```python
from build123d import *

# Parameters (mm, degrees)
SKETCH1_R           = 75
BOSS_EXTRUDE1_DEPTH = 102
SKETCH3_R           = 51
BOSS_EXTRUDE2_DEPTH = 102
SKETCH4_R           = 38
BOSS_EXTRUDE3_DEPTH = 75


with BuildPart() as part:
    # Sketch1 → Boss-Extrude1 (new body)
    with BuildSketch(Plane(origin=(0, 0, 0), x_dir=(1, 0, 0), z_dir=(0, 1, 0))):
        with BuildLine():
            Line((-179.614887026, -98.810385884), (-355, 220))
            Line((-355, 220), (-355, 495))
            Line((-355, 495), (355, 495))
            Line((355, 495), (355, 220))
            Line((355, 220), (179.614887026, -98.810385884))
            ThreePointArc((179.614887026, -98.810385884), (0, -205), (-179.614887026, -98.810385884))
        make_face()
        with Locations(Location((0, 0, 0), (0, 0, 270))):
            Circle(SKETCH1_R, mode=Mode.SUBTRACT)
    boss_extrude1 = extrude(amount=BOSS_EXTRUDE1_DEPTH)

    # Sketch3 → Boss-Extrude2 (add)
    with BuildSketch(Plane(origin=(355, 0, 0), x_dir=(0, 0, -1), z_dir=(1, 0, 0))):
        with BuildLine():
            Line((220, 0), (220, 745))
            Line((220, 745), (495, 745))
            Line((495, 745), (901.007583532, 165.230354266))
            ThreePointArc((901.007583532, 165.230354266), (908.13749835, 56.5190099), (815, 0))
            Line((815, 0), (220, 0))
        make_face()
        with Locations((815, 105)):
            Circle(SKETCH3_R, mode=Mode.SUBTRACT)
    boss_extrude2 = extrude(amount=-BOSS_EXTRUDE2_DEPTH)

    # Mirror1: Boss-Extrude2 across plane
    add(boss_extrude2.mirror(Plane(origin=(0, 0, 0), x_dir=(0, 0, 1), z_dir=(1, 0, 0))))

    # Mirror2: Boss-Extrude1 across plane
    add(boss_extrude1.mirror(Plane(origin=(0, 372.5, 0), x_dir=(0, 0, 1), z_dir=(0, -1, 0))))

    # Sketch4 → Boss-Extrude3 (add)
    with BuildSketch(Plane(origin=(100, 0, 0), x_dir=(0, 0, -1), z_dir=(1, 0, 0))):
        with BuildLine():
            Line((440.558080551, 1007.850884872), (220, 745))
            Line((220, 745), (454.97331208, 745))
            Line((454.97331208, 745), (578.446080312, 892.149115128))
            ThreePointArc((578.446080312, 892.149115128), (567.352965303, 1018.943999881), (440.558080551, 1007.850884872))
        make_face()
        with Locations((509.502080431, 950)):
            Circle(SKETCH4_R, mode=Mode.SUBTRACT)
    boss_extrude3 = extrude(amount=BOSS_EXTRUDE3_DEPTH)

    # Mirror3: Boss-Extrude3 across plane
    add(boss_extrude3.mirror(Plane(origin=(0, 0, 0), x_dir=(0, 0, 1), z_dir=(1, 0, 0))))


solid = part.part
```
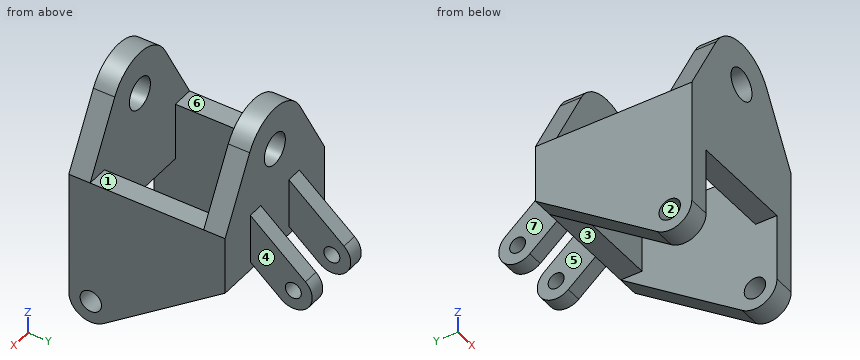
Can you work these out from the model? Positions are in its coordinate system, mm. Face numbers are marked on the shaded views. A direction names the side the tool comes from. Coordinates: 2 decimals unless noted, no trailing zeros. Loops run counter-clockwise (first coordinate to the right, second up) from the corner with the lowest first, then second, coordinate; pieces in that order, holes last. Notation, with made-up numbers: M 45,-20.5 L 66,-20.5 A31 cw 66,11.5 Z; hole C 61.5,63 d6. An arc over 180 degrees is marked long. Put each result on its own line as item: value. Start each with the question number.
(1) I need wall thicknesses on probe 1 along X at (y, z) = (167, -461.5); probe 2 along Y at (x, z) = (81.5, -149.5); probe 3 along X at (y, z) = (916.5, -588.5). Which ranges of each line are inside material? Lowest first, please.
(2) Which directions (+Z, -Z, +X, -X, +Y, -Y) give clear straight access to the entire face, cutting with the end or side of a thin tool? Please do the marked faces 5, 6 and 7.
(3) We'd pull the mould along Z, two halves only. Please class the marked faces 1, 2, 3 and 4: +Z half, -Z half, draft (parallel to the pull), parting line (faces both ways), or undercut.
(4) Imagine slicing it at A-A on x = 0. List the corners of the cut face in (y, z) for me.
(5) Imagine slicing it at C-C on z = -408.5. List the corners of the cut face in (x, y) for me.
(6) Imagine slicing it at D-D on x = -136. List the corners of the cut face in (y, z) for me.
(7) Imagine slicing it at B-B on y = 777.5. List the corners of the cut face in (x, z) for me, and give its area (3 significant figures).
(8) Will these pins go through, and if not, where does the flat tip stop? pin 1 Ø10 at (x, y) = (114.5, 664) entering from -Z; pin 2 Ø5 at (x, z) = (91, -37.5) entering from +Y.
Worked answers:
1. probe 1: x = -355 to -253, 253 to 355
1. probe 2: y = 0 to 102, 643 to 745
1. probe 3: x = -175 to -100, 100 to 175
2. face 5: +Z, -Z, +Y
2. face 6: +Z, +X, -X
2. face 7: +Z, -Z, -X, +Y
3. face 1: +Z half
3. face 2: undercut
3. face 3: -Z half
3. face 4: draft
4. outline: M 0,-495 L 102,-495 L 102,-75 L 0,-75 Z; M 0,75 L 102,75 L 102,205 L 0,205 Z; M 643,-495 L 745,-495 L 745,-75 L 643,-75 Z; M 643,75 L 745,75 L 745,205 L 643,205 Z
5. outline: M -355,0 L 355,0 L 355,745 L 175,745 L 175,969.65 L 100,969.65 L 100,745 L -100,745 L -100,969.65 L -175,969.65 L -175,745 L -355,745 Z; hole M -253,102 L 253,102 L 253,643 L -253,643 Z
6. outline: M 0,-495 L 102,-495 L 102,153.39 L 0,153.39 Z; M 643,-495 L 745,-495 L 745,-454.97 L 892.15,-578.45 A90 ccw 1007.85,-440.56 L 745,-220 L 745,153.39 L 643,153.39 Z; hole C 950,-509.5 d76
7. outline: M -175,-482.24 L -100,-482.24 L -100,-247.27 L -175,-247.27 Z; M 100,-482.24 L 175,-482.24 L 175,-247.27 L 100,-247.27 Z
7. area: 35,200 mm2
8. pin 1: stops at z = -495
8. pin 2: stops at y = 745
